Check sheet for the drawn part. Datum: minimum x, y, z corner. Units: mm. Round coordinates to 2 decimals unless told otherwise and drop trailing zeros. Write each loop counter-clockwise with the first axis right and the second up, starting at its lowest first coordinate (ties: lowest second). Pieces come first, ordered by that corner, then holes.
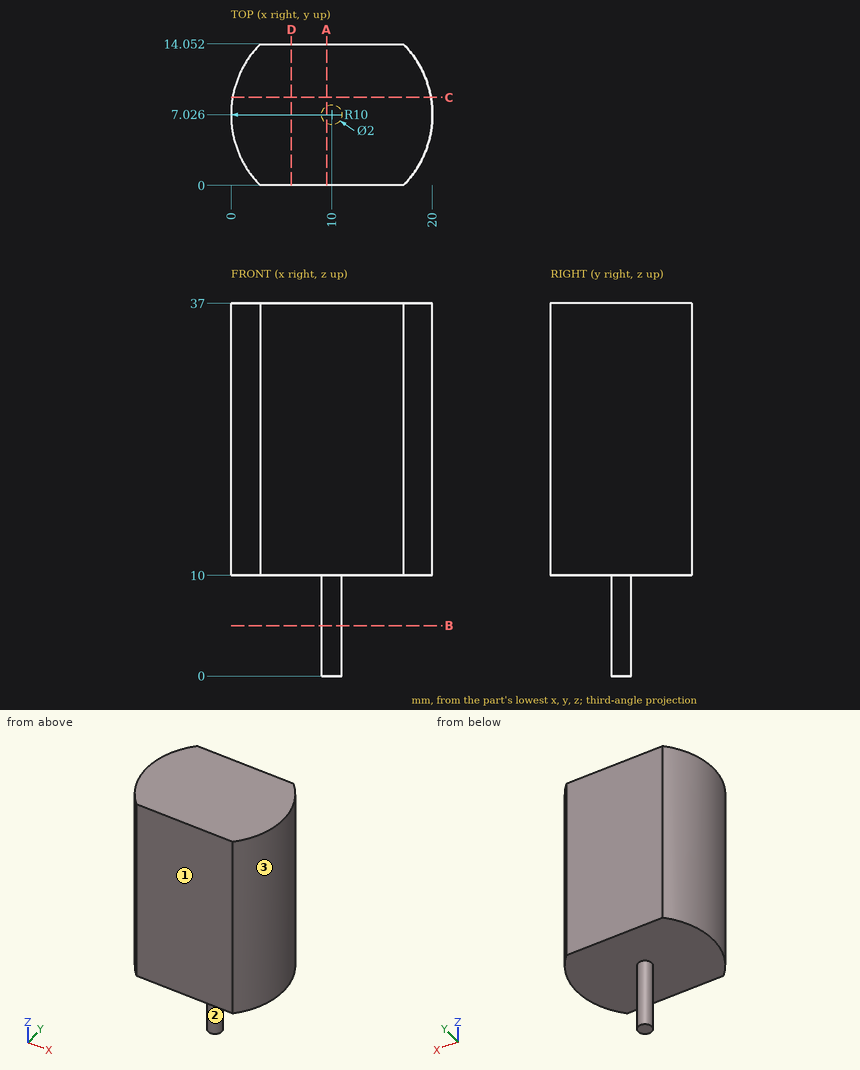
Q1. Sectioned sample at B-B (z = 5). Enter the section's corners in (x, y), plus the area to 3 significant figures.
Recorded:
outline: circle Ø2 at (10, 7.03)
area: 3.14 mm2
Q2. Sectioned sample at A-A (x = 9.5). Enter the section's corners in (y, z), plus the area to 3 significant figures.
Recorded:
outline: (0, 10) - (6.16, 10) - (6.16, 0) - (7.89, 0) - (7.89, 10) - (14.05, 10) - (14.05, 37) - (0, 37) - close
area: 397 mm2
Q3. Material ranges on line 1 along Z through (x, y) = (6.5, 12.25); line 2 along X through (y, z) = (10.5, 19); line 3 along X through (y, z) = (7, 3), recorded low to high.
Recorded:
line 1: z = 10 to 37
line 2: x = 0.62 to 19.38
line 3: x = 9 to 11
Q4. Sectioned sample at D-D (x = 6). Enter the section's corners in (y, z).
Recorded:
outline: (0, 10) - (14.05, 10) - (14.05, 37) - (0, 37) - close
Q5. Release check for a two-part mould opening along X. For the marked faces 1, 2 and 3 record: released by +X, released by -X, zero draft, split by the parting line, or undercut.
Recorded:
face 1: zero draft
face 2: split by the parting line
face 3: released by +X
Q6. Sectioned sample at C-C (y = 8.75). Enter the section's corners in (x, z).
Recorded:
outline: (0.15, 10) - (19.85, 10) - (19.85, 37) - (0.15, 37) - close
Q7. Depth check by flat-ended pin: P1, Ø2, axis at x = 11.5, y = 12, coming from the -Z side; P2, Ø6, axis at y = 3.5, z = 20.5, coming from the +X side; P3, Ø2, axis at x = 6.5, z = 7, coming from the +Y side (1 decimal); P4, Ø4, axis at y = 3.5, z = 21.5, coming from the +X side. Enter the tip coordinate at first touch or a pass-through.
Recorded:
P1: stops at z = 10
P2: stops at x = 19.99
P3: passes through
P4: stops at x = 19.88
